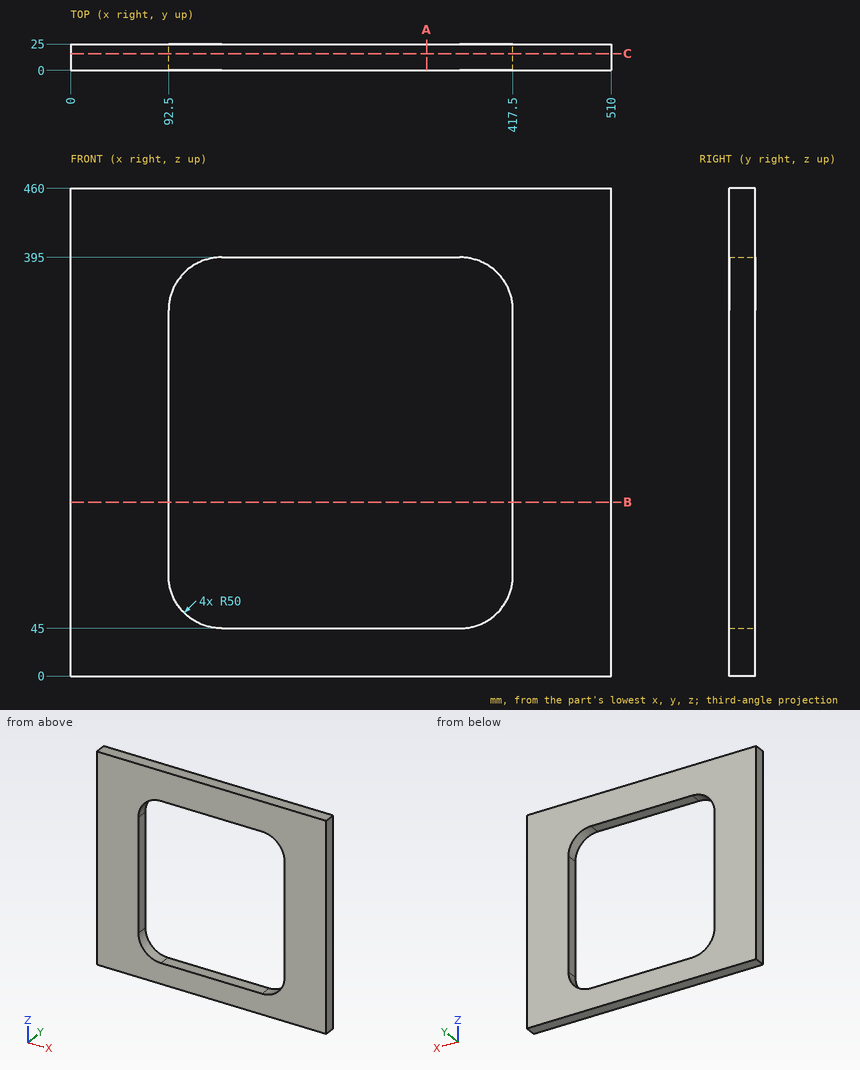
Design review of the part shown in the three views and the two pictorial views. Dimensions are in mm from the part's minimum x, y and z. Round coordinates to 2 decimals unless told otherwise and drop trailing zeros. Write each loop counter-clockwise with the first axis right and the second up, starting at its lowest first coordinate (ties: lowest second). Pieces come first, ordered by that corner, then holes. Notation, with made-up numbers: M 31.5,53 L 60.5,53 A22 ccw 60.5,70 Z; hole C 17.25,41 d11. An arc over 180 degrees is marked long. One line per item, written item: value. Start each with the question number.
1. To check wall thickness, follow probe 1 along Z at (x, y) = (251, 13.5); probe 2 along X at (y, z) = (23.5, 310); probe 3 along Z at (x, y) = (401, 17). State the ranges of each line that lie inside material, in increasing order. Write a range as from..to.
2. Take a section at A-A on x = 336. State the section outline as (y, z) points.
3. Take a section at B-B on z = 164. State the section outline as (x, y) points.
4. Take a section at C-C on y = 16. State the section outline as (x, z) points.
Computed:
1. probe 1: z = 0..45, 395..460
1. probe 2: x = 0..92.5, 417.5..510
1. probe 3: z = 0..57.88, 382.12..460
2. outline: M 0,0 L 25,0 L 25,45 L 0,45 Z; M 0,395 L 25,395 L 25,460 L 0,460 Z
3. outline: M 0,0 L 92.5,0 L 92.5,25 L 0,25 Z; M 417.5,0 L 510,0 L 510,25 L 417.5,25 Z
4. outline: M 0,0 L 510,0 L 510,460 L 0,460 Z; hole M 92.5,95 A50 ccw 142.5,45 L 367.5,45 A50 ccw 417.5,95 L 417.5,345 A50 ccw 367.5,395 L 142.5,395 A50 ccw 92.5,345 Z
